Check sheet for the modelled part. Datum: model origin and axes. Units: mm. Coordinates: 2 decimals unless noted, no trailing zeros. Loops run counter-clockwise (first coordinate to the right, second up) from the corner with the lowest first, then second, coordinate; pieces in that order, holes last. Notation, with made-up numbers: M 24.25,88.25 L 75.25,88.25 A23 cw 75.25,100.25 Z; hole C 53,11 d11. An arc over 180 degrees is marked long. Return JSON: item names as keys, results as strings.
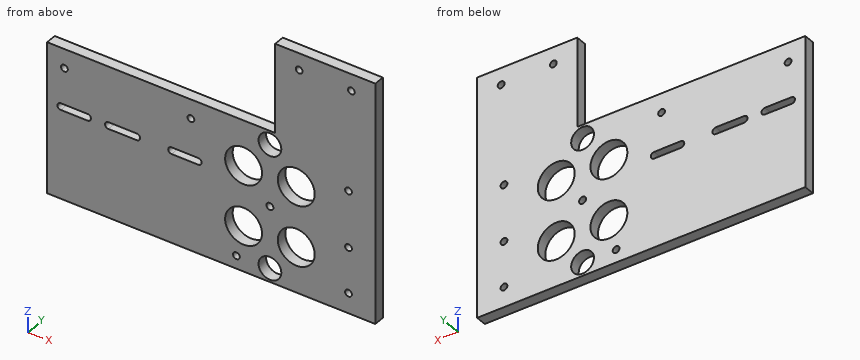
from build123d import *

# Parameters (mm, degrees)
SKETCH1_W                = 88.9
SKETCH1_H                = 80.01
SKETCH1_R                = 9.779
SKETCH1_R_2              = 6.0325
SKETCH1_W_2              = 73.66
SKETCH1_W_3              = 11.43
BOSS_EXTRUDE1_DEPTH      = 5.715
M3_CLEARANCE_HOLE1_D     = 3.6
M3_CLEARANCE_HOLE1_DEPTH = 25.4
M3_CLEARANCE_HOLE1_TIP   = 1.081549114
M3_CLEARANCE_HOLE2_D     = 3.7
M3_CLEARANCE_HOLE2_DEPTH = 25.4
M3_CLEARANCE_HOLE2_TIP   = 1.111592145
CUT_EXTRUDE1_START       = -5.715
CUT_EXTRUDE1_DEPTH       = 5.715


# Read off the part's stored shape, not the designer's step: Cut-Extrude1
with BuildPart() as part:
    # Sketch1 → Boss-Extrude1 (new body)
    # profile 1 of 4: a face of its own
    with BuildSketch(Plane(origin=(0, 0, 0), x_dir=(1, 0, 0), z_dir=(0, 1, 0))):
        Rectangle(SKETCH1_W, SKETCH1_H)
        with Locations(Location((-13.97, -16.002, 0), (0, 0, 270))):
            Circle(SKETCH1_R, mode=Mode.SUBTRACT)
        with Locations(Location((13.97, -16.002, 0), (0, 0, 270))):
            Circle(SKETCH1_R, mode=Mode.SUBTRACT)
        with Locations(Location((-13.97, 16.002, 0), (0, 0, 270))):
            Circle(SKETCH1_R, mode=Mode.SUBTRACT)
        with Locations(Location((13.97, 16.002, 0), (0, 0, 270))):
            Circle(SKETCH1_R, mode=Mode.SUBTRACT)
        with Locations(Location((0, 32.766, 0), (0, 0, 270))):
            Circle(SKETCH1_R_2, mode=Mode.SUBTRACT)
        with Locations(Location((0, -32.766, 0), (0, 0, 270))):
            Circle(SKETCH1_R_2, mode=Mode.SUBTRACT)
    # profile 2 of 4: a face of its own
    with BuildSketch(Plane(origin=(0, 0, 0), x_dir=(1, 0, 0), z_dir=(0, 1, 0))):
        with Locations((-81.28, 0)):
            Rectangle(SKETCH1_W_2, SKETCH1_H)
    # profile 3 of 4: a face of its own
    with BuildSketch(Plane(origin=(0, 0, 0), x_dir=(1, 0, 0), z_dir=(0, 1, 0))):
        with Locations((50.165, 0)):
            Rectangle(SKETCH1_W_3, SKETCH1_H)
    # profile 4 of 4: a face of its own
    with BuildSketch(Plane(origin=(0, 0, 0), x_dir=(1, 0, 0), z_dir=(0, 1, 0))):
        Polygon((55.88, -40.005), (44.45, -40.005), (2.794, -40.005), (2.794, -87.249), (55.88, -87.249), align=None)
    extrude(amount=BOSS_EXTRUDE1_DEPTH)

    # M3 Clearance Hole1
    with Locations(Plane(origin=(0, 5.715, 0), x_dir=(1, 0, 0), z_dir=(0, 1, 0))):
        with Locations((-17.78, 33.147), (41.656, 29.337), (41.656, 5.207), (41.656, -24.765), (43.18, -78.359), (15.494, -78.359), (-41.91, -29.845), (-108.966, -29.845)):
            Hole(M3_CLEARANCE_HOLE1_D / 2, depth=M3_CLEARANCE_HOLE1_DEPTH)
            with Locations((0, 0, -(M3_CLEARANCE_HOLE1_DEPTH + M3_CLEARANCE_HOLE1_TIP / 2))):  # 118° drill point
                Cone(0, M3_CLEARANCE_HOLE1_D / 2, M3_CLEARANCE_HOLE1_TIP, mode=Mode.SUBTRACT)

    # M3 Clearance Hole2
    with Locations(Plane(origin=(0, 5.715, 0), x_dir=(1, 0, 0), z_dir=(0, 1, 0))):
        with Locations((0, 0)):
            Hole(M3_CLEARANCE_HOLE2_D / 2, depth=M3_CLEARANCE_HOLE2_DEPTH)
            with Locations((0, 0, -(M3_CLEARANCE_HOLE2_DEPTH + M3_CLEARANCE_HOLE2_TIP / 2))):  # 118° drill point
                Cone(0, M3_CLEARANCE_HOLE2_D / 2, M3_CLEARANCE_HOLE2_TIP, mode=Mode.SUBTRACT)

    # Cut-Extrude1 outline → Cut-Extrude1 (cut)
    with BuildSketch(Plane(origin=(0, 5.715, 0), x_dir=(1, 0, 0), z_dir=(0, 1, 0)).offset(CUT_EXTRUDE1_START)):
        with BuildLine():
            Line((-52.137072336, -10.588243938), (-37.913072336, -10.513831599))
            ThreePointArc((-37.913072336, -10.513831599), (-36.162240737, -8.763), (-37.913072336, -7.012168401))
            Line((-37.913072336, -7.012168401), (-52.137072336, -7.012168401))
            ThreePointArc((-52.137072336, -7.012168401), (-53.925110105, -8.80020617), (-52.137072336, -10.588243938))
        make_face()
        with BuildLine():
            Line((-110.876944468, -10.539089177), (-96.652944596, -10.541))
            ThreePointArc((-96.652944596, -10.541), (-94.874944596, -8.763), (-96.652944596, -6.985))
            Line((-96.652944596, -6.985), (-110.876944468, -6.983089177))
            ThreePointArc((-110.876944468, -6.983089177), (-112.654944468, -8.761089177), (-110.876944468, -10.539089177))
        make_face()
        with BuildLine():
            ThreePointArc((-85.680129902, -6.983089177), (-87.460040724, -8.763), (-85.680129902, -10.542910823))
            Line((-85.680129902, -10.542910823), (-70.60161816, -10.542910823))
            ThreePointArc((-70.60161816, -10.542910823), (-68.821707338, -8.763), (-70.60161816, -6.983089177))
            Line((-70.60161816, -6.983089177), (-85.680129902, -6.983089177))
        make_face()
    extrude(amount=CUT_EXTRUDE1_DEPTH, mode=Mode.SUBTRACT)


solid = part.part
1) Section check B-B on z = 0. Record the cut outline in (x, y) (3 decimals).
Answers:
{"outline": "M -118.11,0 L -1.85,0 L -1.85,5.715 L -118.11,5.715 Z; M 1.85,0 L 55.88,0 L 55.88,5.715 L 1.85,5.715 Z"}
2) Scan lines: line 1 along Z through (x, y) = (-76, 2.2) (3 decimals); line 2 along Z through (x, y) = (-52.5, 3.5) (3 decimals); line 3 along Z through (x, y) = (-43, 2.85) (3 decimals). Record each from-to range of solid material in increasing order. Write a range as [from, to].
Answers:
{"line 1": "[-40.005, 6.983], [10.543, 40.005]", "line 2": "[-40.005, 7.049], [10.551, 40.005]", "line 3": "[-40.005, 7.012], [10.54, 28.413], [31.277, 40.005]"}
3) Section check A-A on x = 0. Count the separate pieces of the cut face and the enclosed holes in it, then the cut area to 3 significant figures.
Answers:
{"separate pieces": "4", "enclosed holes": "0", "area": "298 mm²"}
4) Section check D-D on z = 73. Record the cut outline in (x, y) (3 decimals).
Answers:
{"outline": "M 2.794,0 L 55.88,0 L 55.88,5.715 L 2.794,5.715 Z"}
5) Go/stop test with flat-tipped pins: pin 1 Ø1 at (y, z) = (1.5, 45.5) entering from -X; pin 2 Ø3 at (x, y) = (-48, 3) entering from +Z (3 decimals). Record where each tip stops, or that it passes through.
Answers:
{"pin 1": "x = 2.79", "pin 2": "z = 40.005"}
